from build123d import *

# Parameters (mm, degrees)
EXTRUDE_START          = -3.5
SKETCH_1_R             = 8
SKETCH_1_R_2           = 4
EXTRUDE_1_DEPTH        = 7.5
SKETCH_2_R             = 5.5
SKETCH_2_R_2           = 4
EXTRUDE_2_DEPTH        = 0.5
CUT_EXTRUDE_1_DEPTH    = 7.5
HOLE_WIZARD_M4_1_D     = 3.3
HOLE_WIZARD_M4_1_DEPTH = 17.5
HOLE_WIZARD_M4_1_TIP   = 0.991420021


with BuildPart() as part:
    # 草图1 → 凸台-拉伸1 (new body)
    with BuildSketch(Plane.XY.offset(EXTRUDE_START)):
        Circle(SKETCH_1_R)
        Circle(SKETCH_1_R_2, mode=Mode.SUBTRACT)
    extrude(amount=EXTRUDE_1_DEPTH)

    # 草图2 → 凸台-拉伸2 (add)
    with BuildSketch(Plane.XY.offset(4)):
        Circle(SKETCH_2_R)
        Circle(SKETCH_2_R_2, mode=Mode.SUBTRACT)
    extrude(amount=EXTRUDE_2_DEPTH)

    # 草图3 → 切除-拉伸1 (cut)
    with BuildSketch(Plane(origin=(0, 0, -3.5), x_dir=(-1, 0, 0), z_dir=(0, 0, -1))):
        with BuildLine():
            Line((-7.858116823, -1.5), (-6, -1.5))
            Line((-6, -1.5), (-6, 1.5))
            Line((-6, 1.5), (-7.858116823, 1.5))
            ThreePointArc((-7.858116823, 1.5), (-8, 0), (-7.858116823, -1.5))
        make_face()
        with BuildLine():
            Line((1.5, -7.858116823), (1.5, -6))
            Line((1.5, -6), (-1.5, -6))
            Line((-1.5, -6), (-1.5, -7.858116823))
            ThreePointArc((-1.5, -7.858116823), (0, -8), (1.5, -7.858116823))
        make_face()
        with BuildLine():
            Line((-1.5, 6), (1.5, 6))
            Line((1.5, 6), (1.5, 7.858116823))
            ThreePointArc((1.5, 7.858116823), (0, 8), (-1.5, 7.858116823))
            Line((-1.5, 7.858116823), (-1.5, 6))
        make_face()
        with BuildLine():
            Line((6, -1.5), (7.858116823, -1.5))
            ThreePointArc((7.858116823, -1.5), (8, 0), (7.858116823, 1.5))
            Line((7.858116823, 1.5), (6, 1.5))
            Line((6, 1.5), (6, -1.5))
        make_face()
    extrude(amount=-CUT_EXTRUDE_1_DEPTH, mode=Mode.SUBTRACT)

    # M4 螺纹孔1
    with Locations(Plane(origin=(5.656854249, -5.656854249, 0), x_dir=(0, 0, -1), z_dir=(0.7071067811865464, -0.7071067811865488, 0))):
        with Locations((0, 0)):
            Hole(HOLE_WIZARD_M4_1_D / 2, depth=HOLE_WIZARD_M4_1_DEPTH)
            with Locations((0, 0, -(HOLE_WIZARD_M4_1_DEPTH + HOLE_WIZARD_M4_1_TIP / 2))):  # 118° drill point
                Cone(0, HOLE_WIZARD_M4_1_D / 2, HOLE_WIZARD_M4_1_TIP, mode=Mode.SUBTRACT)


solid = part.part
The listing builds one solid part. Answer for the finished solid, in the listing's coordinates (mm). A direction names the side the tool comes from. Coordinates: 2 decimals unless noted, no trailing zeros. Order: outer loops, then holes, each group sorted by start corner. A loop starts at its lowest first (then second) coordinate and runs counter-clockwise, first axis right, second up. Notation, with made-up numbers: M 75.25,-25.5 L 86.25,-25.5 A21 cw 86.25,-19.5 Z; hole C 85,68.25 d6. An arc over 180 degrees is marked long. Use CSV: the item, a comma, the result in double quotes.
Q1. Section A-A (y = 0) is taken. Determine the outline of the cut face in (x, z).
Here are the results:
outline,"M -6,-3.5 L -4,-3.5 L -4,4.5 L -5.5,4.5 L -5.5,4 L -6,4 Z; M 4,-3.5 L 6,-3.5 L 6,4 L 5.5,4 L 5.5,4.5 L 4,4.5 Z"
Q2. Straight lines are drawn through the part: L1, parallel to Y at x = 0, z = 2.25; L2, parallel to Z at x = 3.25, y = 7.25; L3, parallel to Z at x = -4.25, y = 5.75. For each, find the intervals that lie inside material, in ascending order.
Here are the results:
L1,"-6 to -4, 4 to 6"
L2,"-3.5 to 4"
L3,"-3.5 to -1.26, 1.26 to 4"
Q3. Section D-D (z = 3.5) is taken. Determine the outline of the cut face in (x, y).
Here are the results:
outline,"M -7.86,-1.5 A8 ccw -1.5,-7.86 L -1.5,-6 L 1.5,-6 L 1.5,-7.86 A8 ccw 7.86,-1.5 L 6,-1.5 L 6,1.5 L 7.86,1.5 A8 ccw 1.5,7.86 L 1.5,6 L -1.5,6 L -1.5,7.86 A8 ccw -7.86,1.5 L -6,1.5 L -6,-1.5 Z; hole C 0,0 d8"
Q4. A tool of negligible diameter and unlimited length cuts with its end or side. For faces 1 (the flat face through (7, 1.5, 0)), 2 (the flat face through (-7, -1.5, 0)), 3 (the flat face through (1.5, -7, 0)), from which of +Z, -Z, +X, -X, +Y, -Y can it reach the whole face along a straight path? Write none if from no direction.
Here are the results:
face 1,"+Z, -Z, +X"
face 2,"+Z, -Z, -X"
face 3,"+Z, -Z, -Y"
Q5. Given pin 1 Ø1.5 at (x, z) = (6, -2) entering from +Y; pin 2 Ø0.9 at (y, z) = (7, 0.5) entering from -X; pin 3 Ø0.6 at (x, z) = (7, 0) entering from +Y; pin 4 Ø2 at (x, z) = (-2, -1.5) entering from -Y, each flat-ended and moving along its own axis, determine where each tip first touches the part or whether it passes through.
Here are the results:
pin 1,"y = 6.04"
pin 2,"x = -4.51"
pin 3,"y = 4.37"
pin 4,"y = -7.86"
Q6. Section B-B (z = -0.25) is taken. Determine the outline of the cut face in (x, y), then the cut area to 3 significant figures.
Here are the results:
outline,"M -7.86,-1.5 A8 ccw -1.5,-7.86 L -1.5,-6 L 1.5,-6 L 1.5,-7.86 A8 ccw 4.38,-6.69 L 1.43,-3.74 A4 cw -3.74,1.43 L -6.69,4.38 A8 ccw -7.86,1.5 L -6,1.5 L -6,-1.5 Z; M -4.38,6.69 L -1.43,3.74 A4 cw 3.74,-1.43 L 6.69,-4.38 A8 ccw 7.86,-1.5 L 6,-1.5 L 6,1.5 L 7.86,1.5 A8 ccw 1.5,7.86 L 1.5,6 L -1.5,6 L -1.5,7.86 A8 ccw Z"
area,"101 mm2"
Q7. Determine the mould class of faces 4 (the flat face through (-1.5, -7, 0)), 5 (the cylindrical face through (5.704, 5.609, 0.197)), 6 (the flat face through (-7, 1.5, 0)), 7 (the flat face through (6, 0, 0)) for opening direction Y: pulls with the +Y half, pulls with the -Y half, needs draft (parallel to the pull), parting line crosses it, or undercut.
Here are the results:
face 4,"needs draft"
face 5,"pulls with the +Y half"
face 6,"undercut"
face 7,"undercut"
